Here's the drawing with two shaded views (mm, measured from the low corner). I have some questions. A direction names the side the tool comes from. Give positions to 0.01 mm unless a question says otherwise; leave off trailing zeros. Write each loop counter-clockwise with the first axis right and the second up, starting at its lowest first coordinate (ties: lowest second). Pieces come first, ordered by that corner, then holes. Notation, with made-up numbers: (10.5, 8.5) - (69.5, 8.5) arc R13 ccw to (69.5, 29.5) - close; hole circle Ø9 at (16.25, 76). An arc over 180 degrees is marked (long way). Write item = value, one per line.
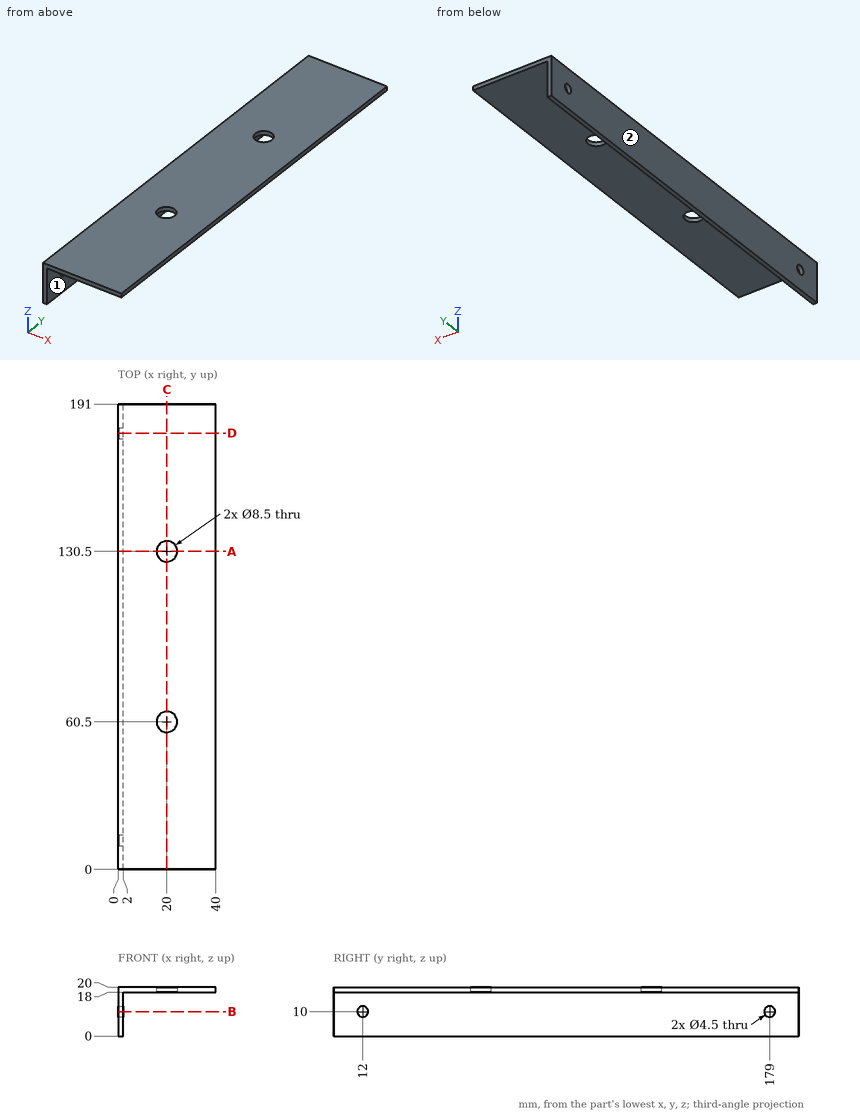
1. If we section it at B-B, the plane z = 10: Please give me the cut outline in (x, y), and give its area (3 significant figures).
Filled sheet:
outline = (0, 0) - (2, 0) - (2, 9.75) - (0, 9.75) - close; (0, 14.25) - (2, 14.25) - (2, 176.75) - (0, 176.75) - close; (0, 181.25) - (2, 181.25) - (2, 191) - (0, 191) - close
area = 364 mm2
2. For pin 1 (10 mm diameter, centred on y = 101, z = 6, fed in from +X); pin 2 (13.5 mm diameter, centred on x = 20, y = 60.5, fed in from -Z), each with a flat end and sliding along its axis, tell me the tip position at first contact or that it passes through.
Filled sheet:
pin_1 = 2
pin_2 = 18
3. If we section it at A-A, the plane y = 130.5: Please give me the cut outline in (x, z).
Filled sheet:
outline = (0, 0) - (2, 0) - (2, 18) - (15.75, 18) - (15.75, 20) - (0, 20) - close; (24.25, 18) - (40, 18) - (40, 20) - (24.25, 20) - close
4. Which directions (+Z, -Z, +X, -X, +Y, -Y) give clear straight access to the entire face, cutting with the end or side of a thin tool? Please do the marked faces 1 and 2.
Filled sheet:
face_1 = -Z, +X, +Y, -Y
face_2 = +Z, -Z, -X, +Y, -Y
5. If we section it at D-D, the plane y = 179: Please give me the cut outline in (x, z).
Filled sheet:
outline = (0, 0) - (2, 0) - (2, 7.75) - (0, 7.75) - close; (0, 12.25) - (2, 12.25) - (2, 18) - (40, 18) - (40, 20) - (0, 20) - close
6. If we section it at C-C, the plane x = 20: Please give me the cut outline in (y, z), and give its area (3 significant figures).
Filled sheet:
outline = (0, 18) - (56.25, 18) - (56.25, 20) - (0, 20) - close; (64.75, 18) - (126.25, 18) - (126.25, 20) - (64.75, 20) - close; (134.75, 18) - (191, 18) - (191, 20) - (134.75, 20) - close
area = 348 mm2
7. I need wall thicknesses on line 1 (Y direction, x = 20, z = 19.4); line 2 (Y direction, x = 1.4, z = 10); line 3 (Z direction, x = 26.5, y = 131). Which ranges of each line are inside material? Lowest first, please.
Filled sheet:
line_1 = 0 to 56.25, 64.75 to 126.25, 134.75 to 191
line_2 = 0 to 9.75, 14.25 to 176.75, 181.25 to 191
line_3 = 18 to 20
